The listing builds one solid part. Answer for the finished solid, in the listing's coordinates (mm). Give positions to 0.01 mm unless a question says otherwise; leave off trailing zeros. Write each loop counter-clockwise with the first axis right and the second up, starting at its lowest first coordinate (ties: lowest second). Pieces come first, ordered by that corner, then holes. Notation, with made-up numbers: (-39.5, 37) - (-4.5, 37) arc R33 ccw to (-4.5, 65) - close; hole circle Ø11 at (-1.75, -2.5). An arc over 180 degrees is marked (long way). Answer in a Markdown table with one row per item. Add a question column.
from build123d import *

# Parameters (mm, degrees)
F0_R      = 25.4
F1_DEPTH  = 3
F1_FACE_R = 25.4
F2_DEPTH  = 2.54
F2_TAPER  = -45
F5_R      = 20.955
F6_DEPTH  = 11.081
F7_SIZE   = 2.54


# Not quite as in the source:
# - a fillet or chamfer that OpenCascade refuses, or shapes differently, is made with other operations: its cross-section is extruded or revolved along the edge and cut away or added


with BuildPart() as f1:
    # F0 (on Top) → F1 (new body)
    with BuildSketch(Plane.XY):
        Circle(F0_R)
    extrude(amount=F1_DEPTH)

    # F1_face (on face) → F2 (join)
    with BuildSketch(Plane.XY.offset(3)):
        Circle(F1_FACE_R)
    extrude(amount=F2_DEPTH, taper=F2_TAPER)

    # F3: F1 across plane


with BuildPart() as f1_1:
    add(f1.part)
    add(f1.part.mirror(Plane.XY))

    # F4: chamfer of 1.27 on 2 edges, made by hand

    # F4_s1 → F4_t2 (revolve, cut)
    with BuildSketch(Plane.XZ):
        Polygon((27.0419743879, 4.6419743879), (26.67, 5.54), (27.94, 5.54), align=None)
    revolve(axis=Axis((0, 0, 5.54), (0, 0, -1)), mode=Mode.SUBTRACT)

    # F4_s3 → F4_t4 (revolve, cut)
    with BuildSketch(Plane.XZ):
        Polygon((27.0419743879, -4.6419743879), (26.67, -5.54), (27.94, -5.54), align=None)
    revolve(axis=Axis((0, 0, -5.54), (0, 0, -1)), mode=Mode.SUBTRACT)

    # F5 (on face) → F6 (cut, through all)
    with BuildSketch(Plane(origin=(0, 0, -5.54), x_dir=(1, 0, 0), z_dir=(0, 0, -1))):
        Circle(F5_R)
    extrude(amount=-F6_DEPTH, mode=Mode.SUBTRACT)

    # F7
    f7_edges = [f1_1.edges().sort_by_distance(p)[0] for p in [
        (-20.955, 0, 5.54),
        (-20.955, 0, -5.54),
    ]]
    chamfer(f7_edges, length=F7_SIZE)


solid = f1_1.part
1. Section B-B (z = -1.5) is taken. Give the vertices of the cut face in (x, y) (3 decimals), and give its area (3 significant figures).
2. Straight lines are drawn through the part: L1, parallel to Y at x = 0, z = -1.3 (3 decimals); L2, parallel to X at y = 8, z = -2; L3, parallel to X at y = 13, z = 0.5. For each, find the intervals that lie inside material, in ascending order. Write a range as [from, to].
3. The mould has two halves that part along Y. Classify faces 1 (the face through (-5.506, -24.796, 0.042)), 2 (the face through (-2.728, -20.777, -0.042)), 3 (the face through (0, -24, -5.54)): +Y half, -Y half, draft (parallel to the pull), parting line (faces both ways), or undercut.
4. Section A-A (x = 0) is taken. Give the vertices of the cut face in (y, z) (3 decimals), and give its area (3 significant figures).
5. Given pin 1 Ø4 at (x, z) = (3.5, 0) entering from +Y; pin 2 Ø2 at (x, z) = (10, 2) entering from -Y; pin 3 Ø1 at (y, z) = (-16.5, -2.5) entering from -X, each flat-ended and moving along its own axis, determine where each tip first touches the part or whether it passes through.
Geometry check:
| question | item | result |
|---|---|---|
| 1 | outline | circle Ø50.8 at (0, 0); hole circle Ø41.91 at (0, 0) |
| 1 | area | 647 mm² |
| 2 | L1 | [-25.4, -20.955], [20.955, 25.4] |
| 2 | L2 | [-24.11, -19.37], [19.37, 24.11] |
| 2 | L3 | [-21.82, -16.44], [16.44, 21.82] |
| 3 | face 1 | parting line |
| 3 | face 2 | undercut |
| 3 | face 3 | draft |
| 4 | outline | (-27.042, -4.642) - (-26.67, -5.54) - (-23.495, -5.54) - (-20.955, -3) - (-20.955, 3) - (-23.495, 5.54) - (-26.67, 5.54) - (-27.042, 4.642) - (-25.4, 3) - (-25.4, -3) - close; (20.955, -3) - (23.495, -5.54) - (26.67, -5.54) - (27.042, -4.642) - (25.4, -3) - (25.4, 3) - (27.042, 4.642) - (26.67, 5.54) - (23.495, 5.54) - (20.955, 3) - close |
| 4 | area | 96.2 mm² |
| 5 | pin 1 | y = 25.36 |
| 5 | pin 2 | y = -23.75 |
| 5 | pin 3 | x = -19.73 |
